Geometry: see drawing. Coordinates: mm, zero at the bounding-box minimum. Coordinates: 2 decimals unless noted, no trailing zeros. Loops run counter-clockwise (first coordinate to the right, second up) from the corner with the lowest first, then second, coordinate; pieces in that order, holes last. Notation, with made-up numbers: (20.25, 47) -> (58.25, 47) arc R13 ccw to (58.25, 66) -> close; hole circle Ø11 at (71, -4.75). An arc over 180 degrees is marked (long way). Answer as a JSON object with one key per item and string values.
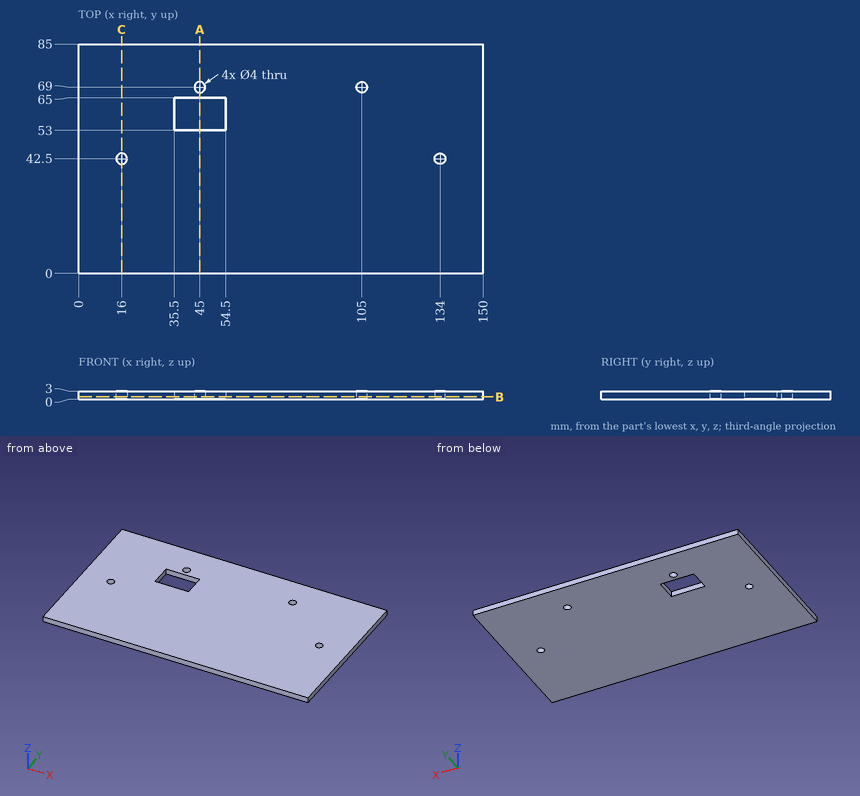
1. Section query C-C (x = 16). Return loops of the section in (y, z), plus the area to 3 significant figures.
Reply:
{"outline": "(0, 0) -> (40.5, 0) -> (40.5, 3) -> (0, 3) -> close; (44.5, 0) -> (85, 0) -> (85, 3) -> (44.5, 3) -> close", "area": "243 mm2"}
2. Line query: line 1 along X through (y, z) = (69, 1); line 2 along X through (y, z) = (63, 2); line 3 along Y through (x, z) = (45, 1.4). Output: solid intervals per line, ascending.
Reply:
{"line 1": "x = 0 to 43, 47 to 103, 107 to 150", "line 2": "x = 0 to 35.5, 54.5 to 150", "line 3": "y = 0 to 53, 65 to 67, 71 to 85"}
3. Section query A-A (x = 45). Return loops of the section in (y, z), plus the area to 3 significant figures.
Reply:
{"outline": "(0, 0) -> (53, 0) -> (53, 3) -> (0, 3) -> close; (65, 0) -> (67, 0) -> (67, 3) -> (65, 3) -> close; (71, 0) -> (85, 0) -> (85, 3) -> (71, 3) -> close", "area": "207 mm2"}
4. Section query B-B (z = 0.9). Return loops of the section in (x, y).
Reply:
{"outline": "(0, 0) -> (150, 0) -> (150, 85) -> (0, 85) -> close; hole circle Ø4 at (16, 42.5); hole (35.5, 53) -> (54.5, 53) -> (54.5, 65) -> (35.5, 65) -> close; hole circle Ø4 at (45, 69); hole circle Ø4 at (105, 69); hole circle Ø4 at (134, 42.5)"}
